Geometry check sheet. Reference: the model listing, model coordinates, mm. Round coordinates to 2 decimals unless told otherwise and drop trailing zeros. Order: outer loops, then holes, each group sorted by start corner. A loop starts at its lowest first (then second) coordinate and runs counter-clockwise, first axis right, second up.
(1) Cross-section at A-A on x = -4.5. Enter the section's corners in (y, z).
(2) Cross-section at C-C on y = 0.05. Enter the section's corners in (x, z), and give its area (3 significant figures).
(3) Cross-section at D-D on x = -12.5. Enter the section's corners in (y, z), and give its area (3 significant figures).
(4) Thickness scan on L1, parallel to X at y = 0.05, z = 0; L2, parallel to Z at x = 8, y = 0.05; L3, parallel to Z at x = -3.5, y = 0.05. Record the ranges inside material, lowest first.
(5) Cross-section at B-B on z = 0. Enter the section's corners in (x, y).
from build123d import *

# Parameters (mm, degrees)
SKETCH26_R          = 11.35
BOSS_EXTRUDE1_DEPTH = 0.096


with BuildPart() as part:
    # Sketch26 → Boss-Extrude1 (new body)
    with BuildSketch(Plane(origin=(0, 0, 0), x_dir=(-1, 0, 0), z_dir=(0, 1, 0))):
        with BuildLine():
            Line((-17.412906679, 6.337779723), (-15.005687805, 5.461623706))
            ThreePointArc((-15.005687805, 5.461623706), (-14.455056516, 4.972678709), (-14.388476201, 4.239310392))
            ThreePointArc((-14.388476201, 4.239310392), (-12.012278216, -8.983605738), (0, -15))
            ThreePointArc((0, -15), (12.012278216, -8.983605738), (14.388476201, 4.239310392))
            ThreePointArc((14.388476201, 4.239310392), (14.455056516, 4.972678709), (15.005687805, 5.461623706))
            Line((15.005687805, 5.461623706), (17.412906679, 6.337779723))
            ThreePointArc((17.412906679, 6.337779723), (19.324147584, 8.250755696), (19.084800719, 10.944272346))
            ThreePointArc((19.084800719, 10.944272346), (16.129508637, 17.491581777), (14.553727529, 24.5))
            Line((14.553727529, 24.5), (8.5, 24.5))
            Line((8.5, 24.5), (8.5, 22))
            ThreePointArc((8.5, 22), (8.060660172, 20.939339828), (7, 20.5))
            Line((7, 20.5), (-7, 20.5))
            ThreePointArc((-7, 20.5), (-8.060660172, 20.939339828), (-8.5, 22))
            Line((-8.5, 22), (-8.5, 24.5))
            Line((-8.5, 24.5), (-14.553727529, 24.5))
            ThreePointArc((-14.553727529, 24.5), (-16.129508637, 17.491581777), (-19.084800719, 10.944272346))
            ThreePointArc((-19.084800719, 10.944272346), (-19.324147584, 8.250755696), (-17.412906679, 6.337779723))
        make_face()
        with Locations(Location((0, 0, 0), (0, 0, 90))):
            Circle(SKETCH26_R, mode=Mode.SUBTRACT)
    extrude(amount=BOSS_EXTRUDE1_DEPTH)


solid = part.part
Found:
1. outline: (0, -14.31) - (0.1, -14.31) - (0.1, -10.42) - (0, -10.42) - close; (0, 10.42) - (0.1, 10.42) - (0.1, 20.5) - (0, 20.5) - close
2. outline: (-19.08, 10.94) arc R3.2 ccw to (-17.41, 6.34) - (-15.01, 5.46) arc R1 cw to (-14.39, 4.24) arc R15 ccw (long way) to (14.39, 4.24) arc R1 cw to (15.01, 5.46) - (17.41, 6.34) arc R3.2 ccw to (19.08, 10.94) arc R35.48 cw to (14.55, 24.5) - (8.5, 24.5) - (8.5, 22) arc R1.5 cw to (7, 20.5) - (-7, 20.5) arc R1.5 cw to (-8.5, 22) - (-8.5, 24.5) - (-14.55, 24.5) arc R35.48 cw to start; hole circle Ø22.7 at (0, 0)
2. area: 689 mm2
3. outline: (0, -8.29) - (0.1, -8.29) - (0.1, 24.5) - (0, 24.5) - close
3. area: 3.15 mm2
4. L1: x = -15 to -11.35, 11.35 to 15
4. L2: z = -12.69 to -8.05, 8.05 to 20.88
4. L3: z = -14.59 to -10.8, 10.8 to 20.5
5. outline: (-15, 0) - (-11.35, 0) - (-11.35, 0.1) - (-15, 0.1) - close; (11.35, 0) - (15, 0) - (15, 0.1) - (11.35, 0.1) - close
